from build123d import *

# Parameters (mm, degrees)
F0_R     = 31.0947263036
F1_DEPTH = 89.0598669648
F3_DEPTH = 37.2095629573
F5_DEPTH = 51.1443465948


with BuildPart() as f1:
    # F0 (on Front) → F1 (new body)
    with BuildSketch(Plane.XZ):
        Circle(F0_R)
    extrude(amount=F1_DEPTH)

    # F2 (on face) → F3 (cut)
    with BuildSketch(Plane.XZ.offset(89.0598669648)):
        with BuildLine():
            Line((-10.8266547322, -29.1490231604), (-10.8266547322, 0))
            Line((-10.8266547322, 0), (-10.8266547322, 29.1490231604))
            ThreePointArc((-10.8266547322, 29.1490231604), (-31.0947263036, 0), (-10.8266547322, -29.1490231604))
        make_face()
    extrude(amount=-F3_DEPTH, mode=Mode.SUBTRACT)

    # F4 (on face) → F5 (cut)
    with BuildSketch(Plane.XZ.offset(51.8503040075)):
        with BuildLine():
            Line((-10.8266547322, -28.2442569733), (-10.8266547322, 27.0338580012))
            ThreePointArc((-10.8266547322, 27.0338580012), (-30.3341260618, -0.605199486), (-10.8266547322, -28.2442569733))
        make_face()
    extrude(amount=-F5_DEPTH, mode=Mode.SUBTRACT)


solid = f1.part
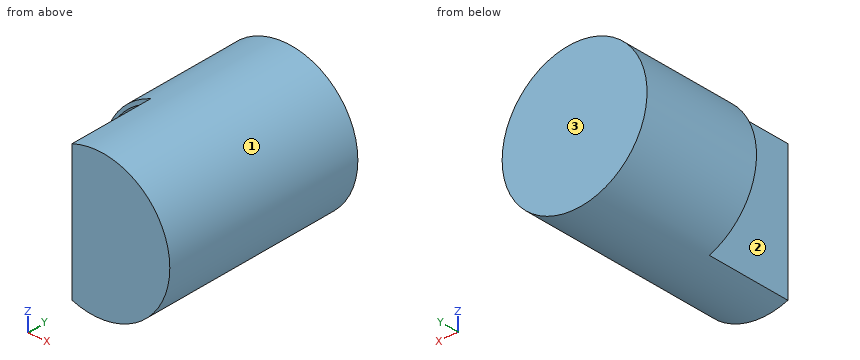
Design review of the part built by this model. Coordinates are the model's own, in mm. Face numbers are marked on the shaded views. Give positions to 0.01 mm unless a question says otherwise; leave off trailing zeros. Write each loop counter-clockwise with the first axis right and the second up, starting at its lowest first coordinate (ties: lowest second). Pieces come first, ordered by that corner, then holes. Notation, with made-up numbers: M -37.75,44.25 L -29.75,44.25 A22 ccw -29.75,69.25 Z; hole C -1,23 d8. An arc over 180 degrees is marked long. Answer as a JSON object with one key per item and string values. Group by question number.
1) For line 1 along Y through (x, z) = (-12, 21.5); line 2 along Z through (x, y) = (-11, -43.5); line 3 along X through (y, z) = (-16, -10), list the stretches that pass through material, from the lowest coordinate up.
2) Mouldability with a two-part tool opening along X and no side actions: class the marked faces 1, 2 and 3 as released by +X, released by -X, zero draft, split by the parting line, or undercut.
3) We need section B-B (y = -45.5). Give the boundary of the cut face in (x, z).
4) Clearance check with flat-ended pins moving along their axes: pin 1 Ø6 at (x, y) = (-16.5, -35) entering from -Z; pin 2 Ø6 at (x, y) = (-8, -66) entering from -Z; pin 3 Ø4 at (x, y) = (-6, -67) entering from -Z. State where each tip first meets the part, or that it passes through.
5) We need section D-D (z = -18). Give the boundary of the cut face in (x, y).
6) We need section C-C (x = 8). Give the boundary of the cut face in (y, z), and give its area (3 significant figures).
7) We need section A-A (z = 0). Give the boundary of the cut face in (x, y), and give its area (3 significant figures).
Answer key:
{
 "1": {"line 1": "y = -0.71 to 0", "line 2": "z = -29.08 to -28.18, 26.97 to 29.08", "line 3": "x = -29.44 to -28.79, -10.83 to 29.44"},
 "2": {"face 1": "split by the parting line", "face 2": "undercut", "face 3": "zero draft"},
 "3": {"outline": "C 0,0 d62.19; hole M -10.83,-28.24 L -10.83,27.03 A29.33 ccw Z"},
 "4": {"pin 1": "stops at z = -28.01", "pin 2": "stops at z = -30.69", "pin 3": "stops at z = -30.84"},
 "5": {"outline": "M -25.36,-51.85 L -24.62,-51.85 L -24.62,-0.71 L -10.83,-0.71 L -10.83,-89.06 L 25.36,-89.06 L 25.36,0 L -25.36,0 Z"},
 "6": {"outline": "M -89.06,-30.05 L 0,-30.05 L 0,30.05 L -89.06,30.05 Z", "area": "5,350 mm²"},
 "7": {"outline": "M -31.09,-51.85 L -30.33,-51.85 L -30.33,-0.71 L -10.83,-0.71 L -10.83,-89.06 L 31.09,-89.06 L 31.09,0 L -31.09,0 Z", "area": "3,790 mm²"}
}
